Geometry check sheet. Reference: drawing and pictorial views, mm from the part's lowest x, y, z. A direction names the side the tool comes from. Round coordinates to 2 decimals unless told otherwise and drop trailing zeros. Loops run counter-clockwise (first coordinate to the right, second up) from the corner with the lowest first, then second, coordinate; pieces in that order, holes last. Notation, with made-up numbers: (11.25, 16.5) - (43.25, 16.5) arc R17 cw to (43.25, 46.5) - close; hole circle Ø1 at (70.5, 18). An arc over 180 degrees is marked (long way). Answer in a Markdown table with one row per item. Add a question column.
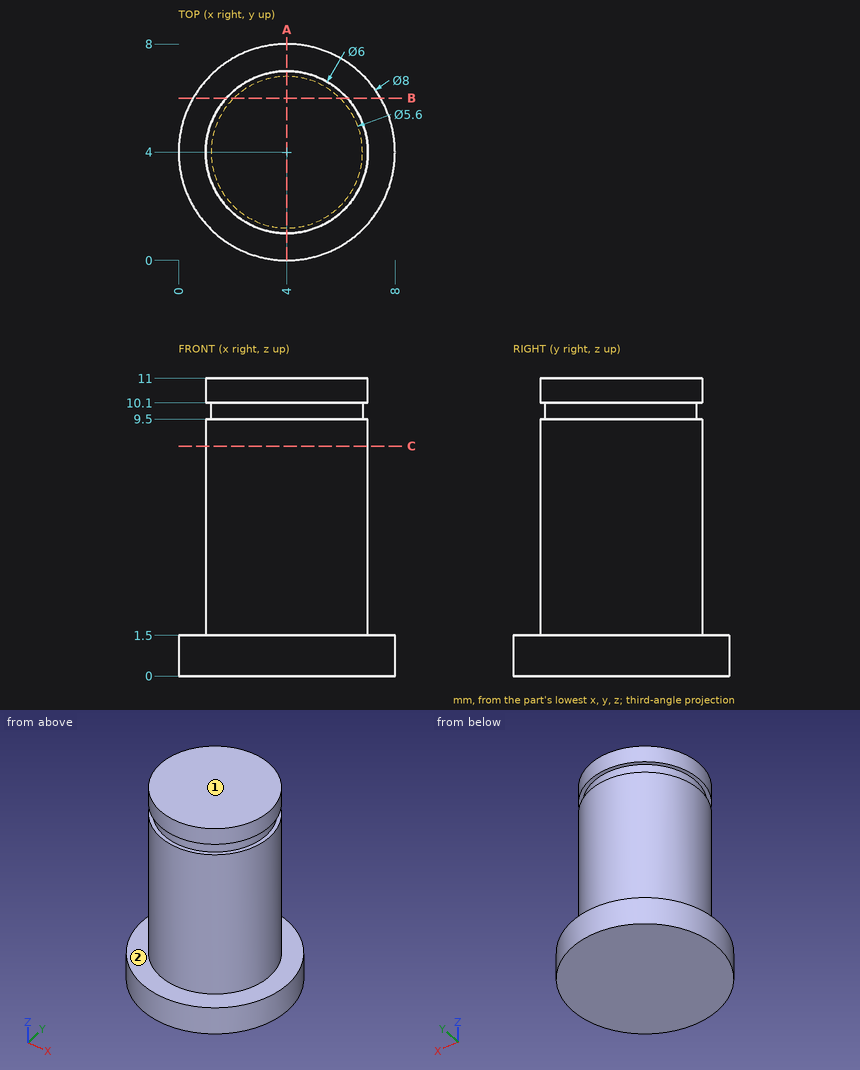
Q1. Cross-section at B-B, the plane y = 6. Enter the section's corners in (x, z), plus the area to 3 significant figures.
Q2. Set-up check for the marked faces 1 and 2: record each of +Z, -Z, +X, -X, +Y, -Y from which the full face is reachable in a straight line by a thin tool's end or side.
Q3. Depth check by flat-ended pin: P1, Ø3, axis at y = 5.5, z = 5.5, coming from the -X side; P2, Ø1, axis at x = 3.5, z = 8.5, coming from the +Y side; P3, Ø1, axis at x = 7, z = 5, coming from the -Y side. Enter the tip coordinate at first touch or a pass-through.
Q4. Scan lines: line 1 (Z direction, x = 0.5, y = 3.5); line 2 (Y direction, x = 1.25, z = 8); line 3 (X direction, y = 0.75, z = 1). Record each from-to range of solid material in increasing order. Write a range as from..to.
Q5. Cross-section at C-C, the plane z = 8.5. Enter the section's corners in (x, y), plus the area to 3 significant figures.
Q6. Cross-section at A-A, the plane x = 4. Enter the section's corners in (y, z), plus the area to 3 significant figures.
Check sheet entries:
| question | item | result |
|---|---|---|
| 1 | outline | (0.54, 0) - (7.46, 0) - (7.46, 1.5) - (6.24, 1.5) - (6.24, 9.5) - (5.96, 9.5) - (5.96, 10.1) - (6.24, 10.1) - (6.24, 11) - (1.76, 11) - (1.76, 10.1) - (2.04, 10.1) - (2.04, 9.5) - (1.76, 9.5) - (1.76, 1.5) - (0.54, 1.5) - close |
| 1 | area | 52.5 mm² |
| 2 | face 1 | +Z, +X, -X, +Y, -Y |
| 2 | face 2 | +Z |
| 3 | P1 | x = 1 |
| 3 | P2 | y = 7 |
| 3 | P3 | y = 2.34 |
| 4 | line 1 | 0..1.5 |
| 4 | line 2 | 2.8..5.2 |
| 4 | line 3 | 1.67..6.33 |
| 5 | outline | circle Ø6 at (4, 4) |
| 5 | area | 28.3 mm² |
| 6 | outline | (0, 0) - (8, 0) - (8, 1.5) - (7, 1.5) - (7, 9.5) - (6.8, 9.5) - (6.8, 10.1) - (7, 10.1) - (7, 11) - (1, 11) - (1, 10.1) - (1.2, 10.1) - (1.2, 9.5) - (1, 9.5) - (1, 1.5) - (0, 1.5) - close |
| 6 | area | 68.8 mm² |
